The listing builds one solid part. Answer for the finished solid, in the listing's coordinates (mm). Face numbers are marked on the shaded views. Give positions to 0.01 mm unless a question says otherwise; leave off trailing zeros. Loops run counter-clockwise (first coordinate to the right, second up) from the corner with the lowest first, then second, coordinate; pieces in that order, holes last. Notation, with made-up numbers: M 80,-36.5 L 139,-36.5 A23 ccw 139,-10.5 Z; hole C 73.25,25.5 d8. An arc over 180 degrees is marked long. Return JSON: item names as keys, results as strings.
from build123d import *

# Parameters (mm, degrees)
SKETCH_2_R          = 14
SKETCH_2_R_2        = 9.6
SKETCH_2_R_3        = 1.6
SKETCH_2_R_4        = 7.5
EXTRUDE_1_DEPTH     = 7
CUT_EXTRUDE_1_DEPTH = 8
SKETCH_5_R          = 14
SKETCH_5_R_2        = 9.6
EXTRUDE_3_DEPTH     = 1
SKETCH_6_R          = 17
SKETCH_6_R_2        = 7.5
SKETCH_6_R_3        = 1.6
EXTRUDE_4_DEPTH     = 1


with BuildPart() as part:
    # 草图2 → 凸台-拉伸1 (new body)
    # profile 1 of 3: a face of its own
    with BuildSketch(Plane(origin=(0, 0, 0), x_dir=(1, 0, 0), z_dir=(0, 1, 0))):
        with BuildLine():
            Line((-16.962264151, -1.132075472), (-14, -90))
            ThreePointArc((-14, -90), (0, -76), (14, -90))
            Line((14, -90), (16.962264151, -1.132075472))
            ThreePointArc((16.962264151, -1.132075472), (0, -17), (-16.962264151, -1.132075472))
        make_face()
    # profile 2 of 3: a face of its own
    with BuildSketch(Plane(origin=(0, 0, 0), x_dir=(1, 0, 0), z_dir=(0, 1, 0))):
        with Locations((0, -90)):
            Circle(SKETCH_2_R)
        with Locations(Location((0, -90, 0), (0, 0, 270))):
            Circle(SKETCH_2_R_2, mode=Mode.SUBTRACT)
    # profile 3 of 3: a face of its own
    with BuildSketch(Plane(origin=(0, 0, 0), x_dir=(1, 0, 0), z_dir=(0, 1, 0))):
        with BuildLine():
            Line((-17, 0), (-16.962264151, -1.132075472))
            ThreePointArc((-16.962264151, -1.132075472), (0, -17), (16.962264151, -1.132075472))
            Line((16.962264151, -1.132075472), (17, 0))
            ThreePointArc((17, 0), (0, 17), (-17, 0))
        make_face()
        with Locations(Location((-10.825317547, -6.25, 0), (0, 0, 270))):
            Circle(SKETCH_2_R_3, mode=Mode.SUBTRACT)
        with Locations(Location((-10.825317547, 6.25, 0), (0, 0, 270))):
            Circle(SKETCH_2_R_3, mode=Mode.SUBTRACT)
        with Locations(Location((0, -12.5, 0), (0, 0, 270))):
            Circle(SKETCH_2_R_3, mode=Mode.SUBTRACT)
        with Locations(Location((0, 0, 0), (0, 0, 270))):
            Circle(SKETCH_2_R_4, mode=Mode.SUBTRACT)
        with Locations(Location((0, 12.5, 0), (0, 0, 270))):
            Circle(SKETCH_2_R_3, mode=Mode.SUBTRACT)
        with Locations(Location((10.825317547, -6.25, 0), (0, 0, 270))):
            Circle(SKETCH_2_R_3, mode=Mode.SUBTRACT)
        with Locations(Location((10.825317547, 6.25, 0), (0, 0, 270))):
            Circle(SKETCH_2_R_3, mode=Mode.SUBTRACT)
    extrude(amount=EXTRUDE_1_DEPTH)

    # 草图4 → 切除-拉伸1 (cut)
    with BuildSketch(Plane(origin=(0, 7, 0), x_dir=(1, 0, 0), z_dir=(0, 1, 0))):
        with BuildLine():
            Line((7.5, -26), (7.5, -65))
            ThreePointArc((7.5, -65), (0, -72.5), (-7.5, -65))
            Line((-7.5, -65), (-7.5, -26))
            ThreePointArc((-7.5, -26), (0, -18.5), (7.5, -26))
        make_face()
    extrude(amount=-CUT_EXTRUDE_1_DEPTH, mode=Mode.SUBTRACT)

    # 草图5 → 凸台-拉伸3 (add)
    with BuildSketch(Plane(origin=(0, 7, 0), x_dir=(1, 0, 0), z_dir=(0, 1, 0))):
        with Locations((0, -90)):
            Circle(SKETCH_5_R)
        with Locations(Location((0, -90, 0), (0, 0, 270))):
            Circle(SKETCH_5_R_2, mode=Mode.SUBTRACT)
    extrude(amount=EXTRUDE_3_DEPTH)

    # 草图6 → 凸台-拉伸4 (add)
    with BuildSketch(Plane(origin=(0, 7, 0), x_dir=(1, 0, 0), z_dir=(0, 1, 0))):
        Circle(SKETCH_6_R)
        with Locations(Location((0, 0, 0), (0, 0, 270))):
            Circle(SKETCH_6_R_2, mode=Mode.SUBTRACT)
        with Locations(Location((0, 12.5, 0), (0, 0, 270))):
            Circle(SKETCH_6_R_3, mode=Mode.SUBTRACT)
        with Locations(Location((10.825317547, 6.25, 0), (0, 0, 270))):
            Circle(SKETCH_6_R_3, mode=Mode.SUBTRACT)
        with Locations(Location((10.825317547, -6.25, 0), (0, 0, 270))):
            Circle(SKETCH_6_R_3, mode=Mode.SUBTRACT)
        with Locations(Location((0, -12.5, 0), (0, 0, 270))):
            Circle(SKETCH_6_R_3, mode=Mode.SUBTRACT)
        with Locations(Location((-10.825317547, -6.25, 0), (0, 0, 270))):
            Circle(SKETCH_6_R_3, mode=Mode.SUBTRACT)
        with Locations(Location((-10.825317547, 6.25, 0), (0, 0, 270))):
            Circle(SKETCH_6_R_3, mode=Mode.SUBTRACT)
    extrude(amount=EXTRUDE_4_DEPTH)


solid = part.part
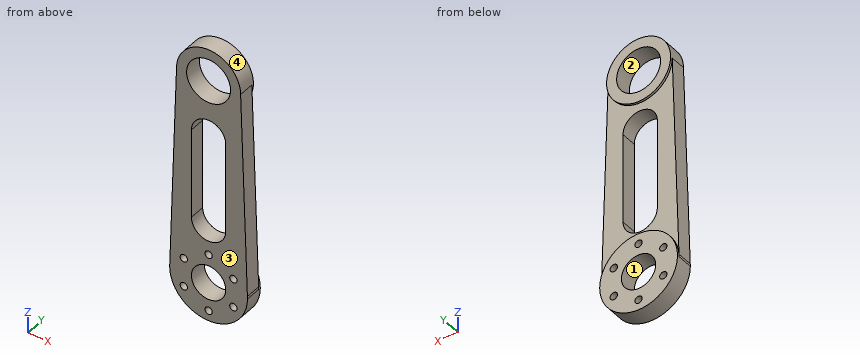
(1) Straight lines are drawn through the part: line 1 along X through (y, z) = (3.25, -6); line 2 along Z through (x, y) = (2, 2.25); line 3 along Z through (x, y) = (5.5, 6). For each, find the intervals that lie inside material, in ascending order.
Values follow:
{"line 1": "-15.91 to -12.41, -9.24 to -4.5, 4.5 to 9.24, 12.41 to 15.91", "line 2": "-16.88 to -7.23, 7.23 to 18.77, 72.23 to 80.61, 99.39 to 103.86", "line 3": "-16.09 to -5.1, 5.1 to 20.9, 70.1 to 82.13, 97.87 to 102.87"}
(2) The part is cut by section D-D (z = 41). Determine the outline of the cut face in (x, y).
Values follow:
{"outline": "M -15.63,0 L -7.5,0 L -7.5,7 L -15.63,7 Z; M 7.5,0 L 15.63,0 L 15.63,7 L 7.5,7 Z"}
(3) Determine the mould class of the marked faces 1, 2, 3 and 4 for opening direction X: released by +X, released by -X, zero draft, split by the parting line, or undercut.
Values follow:
{"face 1": "undercut", "face 2": "undercut", "face 3": "zero draft", "face 4": "split by the parting line"}
(4) The part is cut by section B-B (y = 1.5). Give the number of separate pieces and of enclosed holes in the cut face, and give its area (3 significant figures).
Values follow:
{"separate pieces": "1", "enclosed holes": "9", "area": "2,280 mm²"}
(5) Given pin 1 (5 mm diameter, centred on x = 10.83, z = -6.25, fed in from -Y); pin 2 (1 mm diameter, centred on y = 7, z = 91.5, fed in from -X); pin 3 (3.5 mm diameter, centred on y = 2, z = 44, fed in from +X); pin 4 (2 mm diameter, centred on y = 6, z = -3, fed in from +X), each flat-ended and moving along its own axis, determine where each tip first touches the part or whether it passes through.
Values follow:
{"pin 1": "y = 0", "pin 2": "x = -13.96", "pin 3": "x = 15.59", "pin 4": "x = 16.88"}
(6) The part is cut by section A-A (z = 95). Determine the outline of the cut face in (x, y).
Values follow:
{"outline": "M -13.08,0 L -8.2,0 L -8.2,8 L -13.08,8 Z; M 8.2,0 L 13.08,0 L 13.08,8 L 8.2,8 Z"}
(7) The part is cut by section C-C (z = -6.25). Determine the outline of the cut face in (x, y), and give its area (3 significant figures).
Values follow:
{"outline": "M -15.81,0 L -12.43,0 L -12.43,8 L -15.81,8 Z; M -9.23,0 L -4.15,0 L -4.15,8 L -9.23,8 Z; M 4.15,0 L 9.23,0 L 9.23,8 L 4.15,8 Z; M 12.43,0 L 15.81,0 L 15.81,8 L 12.43,8 Z", "area": "135 mm²"}
